For this review, take the finished solid that the model builds, in its own axes (mm). Face numbers are marked on the shaded views. Round coordinates to 2 decimals unless told otherwise and drop trailing zeros. Write each loop counter-clockwise with the first axis right and the second up, starting at its lowest first coordinate (ties: lowest second). Pieces come first, ordered by that corner, then holes. Notation, with made-up numbers: (81.5, 84.25) -> (111.5, 84.25) arc R18 cw to (111.5, 109.25) -> close; hole circle Ø8 at (16.25, 31). An arc over 180 degrees is marked (long way). Write each question's results on one line, items separated by ' | '. Start each with the question number.
Item 1: Add section B-B (y = 14.5). State the section outline as (x, z) points.
Item 2: Add section A-A (z = -13). State the section outline as (x, y) points.
Item 3: Clearance check with flat-ended pins moving along their axes: pin 1 (10 mm diameter, centred on x = -32.5, y = 4.5, fed in from +Z); pin 2 (4 mm diameter, centred on x = 4.95, z = -8.05, fed in from +Y); pin 3 (8 mm diameter, centred on y = 19.5, z = -70, fed in from +X). State where each tip first meets the part, or that it passes through.
Item 4: The part is to be moulded in two halves that separate along Z. For the marked faces 1 and 2, say which applies: +Z half, -Z half, draft (parallel to the pull), parting line (faces both ways), or undercut.
Item 5: To check wall thickness, follow line 1 along Z through (x, y) = (46, 10.5); line 2 along X through (y, z) = (7.75, 14.5); line 3 along X through (y, z) = (13, -4). State the ranges of each line that lie inside material, in increasing order.
Item 6: Add section C-C (x = 0). State the section outline as (y, z) points.
Item 7: Add section D-D (z = -69.5). State the section outline as (x, y) points, plus the area to 3 significant figures.
from build123d import *

# Parameters (mm, degrees)
EXTRUDE_1_DEPTH          = 3
EXTRUDE_START            = -3.0000001
EXTRUDE_2_OUTLINE_R      = 30
EXTRUDE_2_OUTLINE_R_2    = 28
EXTRUDE_2_DEPTH          = 23.0000001
CUT_EXTRUDE_1_DEPTH      = 120.66431532924713
CUT_EXTRUDE_1_DEPTH_BACK = 120.66431532924713
SKETCH_6_R               = 1.6000000000000003
SKETCH_6_R_2             = 1.5999999999999923
SKETCH_6_R_3             = 1.5999999999999999
SKETCH_6_R_4             = 1.5999999999999257
SKETCH_6_R_5             = 1.6


with BuildPart() as part:
    # 草图1 → 凸台-拉伸1 (new body)
    with BuildSketch(Plane(origin=(0, 0, 0), x_dir=(1, 0, 0), z_dir=(0, 1, 0))):
        with BuildLine():
            Line((69.26629435231834, 24.123359602578955), (22.672692502757357, 79.64558511919181))
            ThreePointArc((22.672692502757354, 79.64558511919181), (-0.2378402213252036, 89.99905718567035), (-22.981333293569364, 79.28362829059616))
            Line((-22.981333293569378, 79.28362829059616), (-69.26729768514315, 24.12216394025026))
            ThreePointArc((-69.26729768514312, 24.122163940250257), (-73.47519800267324, -7.84001220256689), (-46.285964391573756, -25.161464350345888))
            Line((-46.28596439157374, -25.161464350345884), (43.8875404004589, -25.065436701169876))
            ThreePointArc((43.887540400458896, -25.065436701169865), (72.946574545668, -8.916894776595973), (69.26629435231834, 24.12335960257895))
        make_face()
    extrude(amount=EXTRUDE_1_DEPTH)

    # 凸台-拉伸2: read off the stored shape, not the designer's step
    # 凸台-拉伸2 outline → 凸台-拉伸2 (add)
    # profile 1 of 3: a face of its own
    with BuildSketch(Plane(origin=(0, 3, 0), x_dir=(1, 0, 0), z_dir=(0, 1, 0)).offset(EXTRUDE_START)):
        with Locations((-46.285964392, 4.83853565)):
            Circle(EXTRUDE_2_OUTLINE_R)
        with Locations((-46.285964392, 4.83853565)):
            Circle(EXTRUDE_2_OUTLINE_R_2, mode=Mode.SUBTRACT)
    # profile 2 of 3: a face of its own
    with BuildSketch(Plane(origin=(0, 3, 0), x_dir=(1, 0, 0), z_dir=(0, 1, 0)).offset(EXTRUDE_START)):
        with Locations((46.285964392, 4.83853565)):
            Circle(EXTRUDE_2_OUTLINE_R)
        with Locations((46.285964392, 4.83853565)):
            Circle(EXTRUDE_2_OUTLINE_R_2, mode=Mode.SUBTRACT)
    # profile 3 of 3: a face of its own
    with BuildSketch(Plane(origin=(0, 3, 0), x_dir=(1, 0, 0), z_dir=(0, 1, 0)).offset(EXTRUDE_START)):
        with Locations((0, 60)):
            Circle(EXTRUDE_2_OUTLINE_R)
        with Locations((0, 60)):
            Circle(EXTRUDE_2_OUTLINE_R_2, mode=Mode.SUBTRACT)
    extrude(amount=EXTRUDE_2_DEPTH)

    # 草图6 → 切除-拉伸1 (cut, two sides: drawn at the far end of the back side and taken through both)
    with BuildSketch(Plane(origin=(0, 3, 0), x_dir=(1, 0, 0), z_dir=(0, 1, 0)).offset(-CUT_EXTRUDE_1_DEPTH_BACK)):
        with Locations(Location((0, 13, 0), (0, 0, 270))):
            Circle(SKETCH_6_R)
        with Locations(Location((4.9497474683058345, 17.949747468305834, 0), (0, 0, 270))):
            Circle(SKETCH_6_R_2)
        with Locations(Location((4.949747468305964, 8.050252531694156, 0), (0, 0, 270))):
            Circle(SKETCH_6_R_3)
        with Locations(Location((-4.949747468305834, 8.050252531694166, 0), (0, 0, 270))):
            Circle(SKETCH_6_R_4)
        with Locations(Location((-4.949747468305791, 17.949747468305738, 0), (0, 0, 270))):
            Circle(SKETCH_6_R_5)
    extrude(amount=CUT_EXTRUDE_1_DEPTH + CUT_EXTRUDE_1_DEPTH_BACK, mode=Mode.SUBTRACT)


solid = part.part
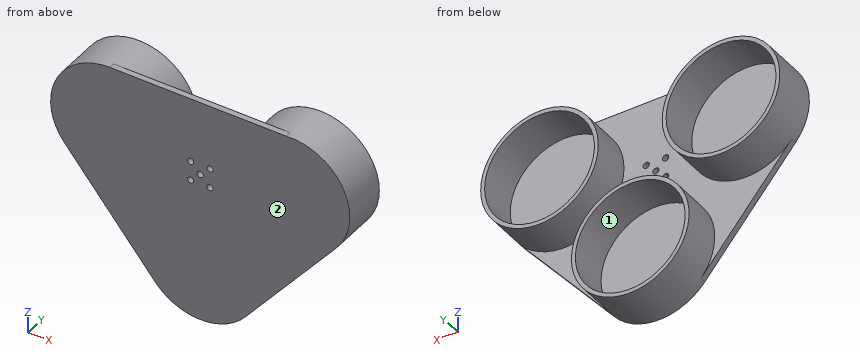
Responses:
1) outline: circle Ø60 at (-46.29, -4.84); circle Ø60 at (0, -60); circle Ø60 at (46.29, -4.84); hole circle Ø56 at (-46.29, -4.84); hole circle Ø56 at (0, -60); hole circle Ø56 at (46.29, -4.84)
2) outline: (-75.15, 0) -> (-1.6, 0) -> (-1.6, 3) -> (-17.42, 3) -> (-17.42, 23) -> (-19.5, 23) -> (-19.5, 3) -> (-73.07, 3) -> (-73.07, 23) -> (-75.15, 23) -> close; (1.6, 0) -> (75.15, 0) -> (75.15, 23) -> (73.07, 23) -> (73.07, 3) -> (19.5, 3) -> (19.5, 23) -> (17.42, 23) -> (17.42, 3) -> (1.6, 3) -> close
3) pin 1: stops at z = 25.15 | pin 2: stops at y = 3 | pin 3: stops at x = 29.39
4) face 1: undercut | face 2: draft
5) line 1: z = -34.84 to -32.84, 23.16 to 25.16 | line 2: x = -69.22 to -66.53, -26.04 to -23.35, 23.35 to 26.04, 66.53 to 69.22 | line 3: x = -76.27 to -74.27, -18.3 to -16.3, 16.3 to 18.3, 74.27 to 76.27
6) outline: (0, -90) -> (23, -90) -> (23, -88) -> (3, -88) -> (3, -32) -> (23, -32) -> (23, -30) -> (3, -30) -> (3, -14.6) -> (0, -14.6) -> close; (0, -11.4) -> (3, -11.4) -> (3, 25.11) -> (0, 25.11) -> close
7) outline: (-31.19, 0) -> (31.19, 0) -> (31.19, 3) -> (28.46, 3) -> (28.46, 23) -> (26.34, 23) -> (26.34, 3) -> (-26.34, 3) -> (-26.34, 23) -> (-28.46, 23) -> (-28.46, 3) -> (-31.19, 3) -> close | area: 272 mm^2
